Autodesk Fusion 360 part; units mm, degrees
sketch "Boceto1" plane through (0, 0, 0) normal (0, 0, 1) x (1, 0, 0)
  line L0 (-24.5, -57.5) -> (24.5, -57.5)
  line L1 (27.5, -54.5) -> (27.5, 54.5)
  line L2 (24.5, 57.5) -> (-24.5, 57.5)
  line L3 (-27.5, 54.5) -> (-27.5, -54.5)
  arc A0 (-24.5, 57.5) -> (-27.5, 54.5) centre (-24.5, 54.5) ccw
  arc A1 (27.5, 54.5) -> (24.5, 57.5) centre (24.5, 54.5) ccw
  arc A2 (-27.5, -54.5) -> (-24.5, -57.5) centre (-24.5, -54.5) ccw
  arc A3 (24.5, -57.5) -> (27.5, -54.5) centre (24.5, -54.5) ccw
  circle A4 centre (-24.5, 54.5) radius 1.5
  circle A5 centre (24.5, 54.5) radius 1.5
  circle A6 centre (-24.5, -54.5) radius 1.5
  circle A7 centre (24.5, -54.5) radius 1.5
  line L4 (21.5, 54.5) -> (-21.5, 54.5)
  line L5 (-27.5, -57.5) -> (-26.9159, -56.2786) construction
  arc A8 (-27.5, -54.5) -> (-24.5, -57.5) centre (-24.5, -54.5) ccw
  arc A9 (-21.5, -54.5) -> (-24.5, -51.5) centre (-24.5, -54.5) ccw
  line L6 (-21.5, -54.5) -> (21.5, -54.5)
  arc A10 (24.5, -57.5) -> (27.5, -54.5) centre (24.5, -54.5) ccw
  arc A11 (24.5, -51.5) -> (21.5, -54.5) centre (24.5, -54.5) ccw
  line L7 (27.5, -57.5) -> (26.9159, -56.2786) construction
  arc A12 (27.5, 54.5) -> (24.5, 57.5) centre (24.5, 54.5) ccw
  arc A13 (21.5, 54.5) -> (24.5, 51.5) centre (24.5, 54.5) ccw
  arc A14 (-24.5, 57.5) -> (-27.5, 54.5) centre (-24.5, 54.5) ccw
  arc A15 (-24.5, 51.5) -> (-21.5, 54.5) centre (-24.5, 54.5) ccw
  circle A16 centre (-24.5, 0) radius 1.5
  line L8 (-24.5, 51.5) -> (-24.5, 3)
  line L9 (-24.5, -3) -> (-24.5, -51.5)
  arc A17 (-24.5, -3) -> (-24.5, 3) centre (-24.5, 0) ccw
  circle A18 centre (24.5, 0) radius 1.5
  line L10 (24.5, -51.5) -> (24.5, -3)
  line L11 (24.5, 3) -> (24.5, 51.5)
  arc A19 (24.5, 3) -> (24.5, -3) centre (24.5, 0) ccw
  dimension "d3" = 3
  dimension "d4" = 3
  dimension "d5" = 3
  dimension "d6" = 3
  dimension "d7" = 6
  dimension "d8" = 6
  dimension "d9" = 6
  dimension "d10" = 6
  dimension "d11" = 3
  dimension "d12" = 3
  dimension "d13" = 3
  dimension "d14" = 3
  dimension "d15" = 6
  dimension "d16" = 3
  dimension "d17" = 6
  dimension "d18" = 3
extrude "Extruir1" add sketch "Boceto1" along normal blind 18
extrude "Extruir2" cut sketch "Boceto1" along normal blind 3 contours L0 L1 L2 L3 A0 A1 A2 A3 A8 A10 A12 A14 | A4 | A5 | A6 | A7 | L4 A9 L6 A11 A13 A15 L8 L9 A17 L10 L11 A19 | A16 | A18
extrude "Extruir3" add sketch "Boceto1" along normal blind 3 contours L0 L1 L2 L3 A0 A1 A2 A3 A8 A10 A12 A14 | A4 | A5 | A6 | A7 | L4 A9 L6 A11 A13 A15 L8 L9 A17 L10 L11 A19 | A16 | A18
fillet "Empalme1" radius 3 1 faces at (-9.1667, 18.1667, 0)
extrude "Extruir4" add 1 faces at (-7.4865, 35.5549, 3) along direction (0, 0, 1) blind 2
Here's how the part is built. I have some questions about the finished solid (model axes, mm). A direction names the side the tool comes from. Coordinates: 2 decimals unless noted, no trailing zeros. Order: outer loops, then holes, each group sorted by start corner. A loop starts at its lowest first (then second) coordinate and runs counter-clockwise, first axis right, second up. Notation, with made-up numbers: M 41,-7 L 54,-7 A15 ccw 54,4 Z; hole C -38.5,64 d4. An arc over 180 degrees is marked long. Answer as a JSON object with one key per item and string values. Group by question number.
(1) Suppose I cut it at A-A, the plane y = 0. Please give me the cut outline in (x, z), then the cut area to 3 significant figures.
(2) If we mould it in two halves opening along Y, with no side actions, what happens to faces 1 (the face through (-26.6, -56.64, 10.4)), 2 (the face through (-22.4, -52.36, 11.41)), 3 (the face through (27.5, -1, 10)), 4 (the face through (-25.7, 55.4, 10.4))? For each: released by +Y, released by -Y, zero draft, split by the parting line, or undercut.
(3) Suppose I cut it at B-B, the plane z = 14. Please give me the cut outline in (x, y), then the cut area to 3 significant figures.
(4) For pin 1 (3 mm diameter, centred on x = 17.5, y = 46, fed in from +Z); pin 2 (1.5 mm diameter, centred on x = 24, y = 0.5, fed in from +Z), each with a flat end and sliding along its axis, tell me the tip position at first contact or that it passes through.
(5) Suppose I cut it at C-C, the plane x = -13.5. Please give me the cut outline in (y, z), then the cut area to 3 significant figures.
(6) I need wall thicknesses on probe 1 along X at (y, z) = (0, 12); probe 2 along Y at (x, z) = (7, 17.25); probe 3 along Y at (x, z) = (-25, 13.5). Which ranges of each line are inside material? Lowest first, please.
(7) Which directions (+Z, -Z, +X, -X, +Y, -Y) give clear straight access to the entire face, cutting with the end or side of a thin tool? Please do faces 5 (the face through (24, 55, 3)), 6 (the face through (26.6, 56.64, 10.4)).
(8) Suppose I cut it at D-D, the plane y = -34. Please give me the cut outline in (x, z).
Values found:
{
 "1": {"outline": "M -27.5,3 A3 ccw -24.5,0 L 24.5,0 A3 ccw 27.5,3 L 27.5,18 L 26,18 L 26,3 L 23,3 L 23,18 L 21.5,18 L 21.5,5 L -21.5,5 L -21.5,18 L -23,18 L -23,3 L -26,3 L -26,18 L -27.5,18 Z", "area": "337 mm^2"},
 "2": {"face 1": "released by -Y", "face 2": "undercut", "face 3": "zero draft", "face 4": "undercut"},
 "3": {"outline": "M -27.5,-54.5 A3 ccw -24.5,-57.5 L 24.5,-57.5 A3 ccw 27.5,-54.5 L 27.5,54.5 A3 ccw 24.5,57.5 L -24.5,57.5 A3 ccw -27.5,54.5 Z; hole C -24.5,-54.5 d3; hole C -24.5,0 d3; hole C -24.5,54.5 d3; hole M -24.5,-51.5 A3 cw -21.5,-54.5 L 21.5,-54.5 A3 cw 24.5,-51.5 L 24.5,-3 A3 cw 24.5,3 L 24.5,51.5 A3 cw 21.5,54.5 L -21.5,54.5 A3 cw -24.5,51.5 L -24.5,3 A3 cw -24.5,-3 Z; hole C 24.5,-54.5 d3; hole C 24.5,0 d3; hole C 24.5,54.5 d3", "area": "990 mm^2"},
 "4": {"pin 1": "stops at z = 5", "pin 2": "stops at z = 3"},
 "5": {"outline": "M -57.5,3 A3 ccw -54.5,0 L 54.5,0 A3 ccw 57.5,3 L 57.5,18 L 54.5,18 L 54.5,5 L -54.5,5 L -54.5,18 L -57.5,18 Z", "area": "649 mm^2"},
 "6": {"probe 1": "x = -27.5 to -26, -23 to -21.5, 21.5 to 23, 26 to 27.5", "probe 2": "y = -57.5 to -54.5, 54.5 to 57.5", "probe 3": "y = -57.46 to -55.91, -53.09 to -1.41, 1.41 to 53.09, 55.91 to 57.46"},
 "7": {"face 5": "+Z", "face 6": "+Z, -Z, +X, +Y"},
 "8": {"outline": "M -27.5,3 A3 ccw -24.5,0 L 24.5,0 A3 ccw 27.5,3 L 27.5,18 L 24.5,18 L 24.5,5 L -24.5,5 L -24.5,18 L -27.5,18 Z"}
}
